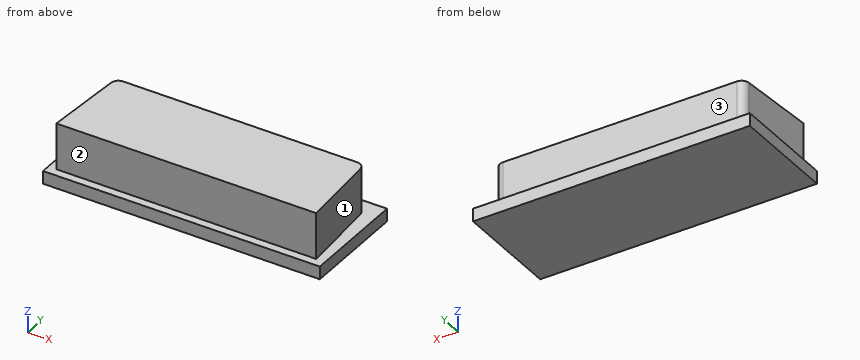
from build123d import *

# Parameters (mm, degrees)
P_IDAT_VYSUNUT_M1_DEPTH = 18
ZAOBLIT1_R              = 3
SKICA2_W                = 107.918638888
SKICA2_H                = 41.380791124
P_IDAT_VYSUNUT_M2_DEPTH = 5


with BuildPart() as part:
    # Skica1 → Přidat vysunutím1 (new body)
    with BuildSketch(Plane.XY):
        Polygon((0, 0), (101.3, 0), (99.05, 33.2), (2.25, 33.2), align=None)
    extrude(amount=P_IDAT_VYSUNUT_M1_DEPTH)

    # Zaoblit1
    zaoblit1_edges = [part.edges().sort_by_distance(p)[0] for p in [
        (2.25, 33.2, 9),
        (99.05, 33.2, 9),
    ]]
    fillet(zaoblit1_edges, radius=ZAOBLIT1_R)

    # Skica2 → Přidat vysunutím2 (add)
    with BuildSketch(Plane(origin=(0, 0, 0), x_dir=(-1, 0, 0), z_dir=(0, 0, -1))):
        with Locations((-50.804022796, 17.445366235)):
            Rectangle(SKICA2_W, SKICA2_H)
    extrude(amount=P_IDAT_VYSUNUT_M2_DEPTH)


solid = part.part
Input: part model. Units: mm. Frame: model coordinates. Face numbers are marked on the shaded views. A direction names the side the tool comes from. Round coordinates to 2 decimals unless told otherwise and drop trailing zeros. Loops run counter-clockwise (first coordinate to the right, second up) from the corner with the lowest first, then second, coordinate; pieces in that order, holes last. Notation, with made-up numbers: M 64.5,26 L 84.5,26 A14 cw 84.5,46 Z; hole C 12,43 d1. An arc over 180 degrees is marked long. Answer as CSV lines item,"result". Start each with the question number.
(1) Section C-C, the plane z = 11.25. Output: boundary loops of the cut face in (x, y).
(2) First-contact query: pin 1 (3 mm diameter, centred on y = 17.5, z = 2.5, fed in from +X); pin 2 (9 mm diameter, centred on x = 58.5, z = 13.5, fed in from +Y); pin 3 (3 mm diameter, centred on x = 9.5, z = 11.5, fed in from -Y). Flat tips, straight axial feed; report the tip coordinate or a pass-through.
(3) Reachability of the marked faces 1, 2 and 3 from +Z, -Z, +X, -X, +Y, -Y: full face, straight path, thin tool, end or side. Return the list, or none.
(4) Line query: line 1 (Y direction, x = 89.5, z = 14.5); line 2 (X direction, y = 12.5, z = 6.5); line 3 (Z direction, x = 21, y = 36). Output: solid intervals per line, ascending. Write a range as [from, to].
(5) Section B-B, the plane y = 12. Output: boundary loops of the cut face in (x, z).
(6) Section A-A, the plane x = 75. Output: boundary loops of the cut face in (y, z).
Values found:
1,outline,"M 0,0 L 101.3,0 L 99.24,30.4 A3 ccw 96.25,33.2 L 5.05,33.2 A3 ccw 2.06,30.4 Z"
2,pin 1,"stops at x = 100.22"
2,pin 2,"stops at y = 33.2"
2,pin 3,"stops at y = 0"
3,face 1,"+Z, +X, +Y"
3,face 2,"+Z, +X, -X, -Y"
3,face 3,"+Z, +X, -X, +Y"
4,line 1,"y = [0, 33.2]"
4,line 2,"x = [0.85, 100.45]"
4,line 3,"z = [-5, 0]"
5,outline,"M -3.16,-5 L 104.76,-5 L 104.76,0 L 100.49,0 L 100.49,18 L 0.81,18 L 0.81,0 L -3.16,0 Z"
6,outline,"M -3.25,-5 L 38.14,-5 L 38.14,0 L 33.2,0 L 33.2,18 L 0,18 L 0,0 L -3.25,0 Z"
